The model under review builds one solid part; all positions refer to its coordinate system, in mm. Face numbers are marked on the shaded views. Coordinates: 2 decimals unless noted, no trailing zeros. Order: outer loops, then holes, each group sorted by start corner. A loop starts at its lowest first (then second) coordinate and runs counter-clockwise, first axis right, second up. Notation, with made-up numbers: M -20.5,0.25 L -1.5,0.25 A32 ccw -1.5,38.25 Z; hole C 22.25,27.5 d5. An arc over 180 degrees is marked long. Answer in a Markdown table with one row per item.
from build123d import *

# Parameters (mm, degrees)
SKETCH1_R           = 3
BOSS_EXTRUDE2_DEPTH = 5


with BuildPart() as part:
    # Sketch1 → Boss-Extrude2 (new body)
    with BuildSketch(Plane(origin=(0, 0, 0), x_dir=(1, 0, 0), z_dir=(0, 1, 0))):
        with BuildLine():
            Line((-107.345005718, 88.870972468), (-6.913400561, -7.225295335))
            ThreePointArc((-6.913400561, -7.225295335), (0.220534203, -9.997567938), (7.225283293, -6.913413146))
            Line((7.225283293, -6.913413146), (99.173678137, 89.182854657))
            ThreePointArc((99.173678137, 89.182854657), (98.86180799, 103.321551097), (84.72311155, 103.009680949))
            Line((84.72311155, 103.009680949), (-0.311882189, 14.138683855))
            Line((-0.311882189, 14.138683855), (-93.518204595, 103.321563138))
            ThreePointArc((-93.518204595, 103.321563138), (-107.656900491, 103.009668365), (-107.345005718, 88.870972468))
        make_face()
        with Locations((-100.431605156, 96.096267803)):
            Circle(SKETCH1_R, mode=Mode.SUBTRACT)
        with Locations((91.948394844, 96.096267803)):
            Circle(SKETCH1_R, mode=Mode.SUBTRACT)
        Circle(SKETCH1_R, mode=Mode.SUBTRACT)
    extrude(amount=BOSS_EXTRUDE2_DEPTH)


solid = part.part
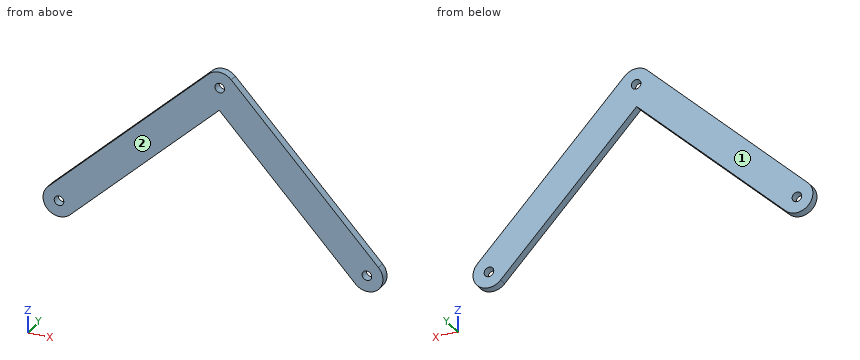
(1) The part is to be moulded in two halves that separate along Y. For the marked faces 1 and 2, say which applies: +Y half, -Y half, draft (parallel to the pull), parting line (faces both ways), or undercut.
Report:
| item | result |
|---|---|
| face 1 | +Y half |
| face 2 | -Y half |
(2) Take a section at C-C (z = -52.5). Write out the cut boundary in (x, y).
Report:
| item | result |
|---|---|
| outline | M -69.33,0 L -40.4,0 L -40.4,5 L -69.33,5 Z; M 36.39,0 L 64.07,0 L 64.07,5 L 36.39,5 Z |
(3) To check wall thickness, follow line 1 (X direction, y = 3.2, z = -98); line 2 (X direction, y = 3.25, z = -53); line 3 (X direction, y = 1.4, z = -59). State the ranges of each line that lie inside material, in increasing order. Write a range as [from, to].
Report:
| item | result |
|---|---|
| line 1 | [-110.25, -102.75], [-98.11, -87.96], [79.93, 89.63], [94.27, 101.77] |
| line 2 | [-69.86, -40.93], [36.87, 64.55] |
| line 3 | [-76.13, -47.2], [42.61, 70.29] |
(4) Take a section at D-D (x = -56.5). Write out the cut boundary in (y, z).
Report:
| item | result |
|---|---|
| outline | M 0,-67.9 L 5,-67.9 L 5,-40.22 L 0,-40.22 Z |
(5) Take a section at A-A (z = 0). Write out the cut boundary in (x, y).
Report:
| item | result |
|---|---|
| outline | M -14.46,0 L -3,0 L -3,5 L -14.46,5 Z; M 3,0 L 13.84,0 L 13.84,5 L 3,5 Z |
(6) Take a section at B-B (y = 2.3). Write out the cut boundary in (x, z) (3 decimals), then the cut area to 3 significant figures.
Report:
| item | result |
|---|---|
| outline | M -107.345,-88.871 A10 ccw -93.518,-103.322 L -0.312,-14.139 L 84.723,-103.01 A10 ccw 99.174,-89.183 L 7.225,6.913 A10 ccw -6.913,7.225 Z; hole C -100.432,-96.096 d6; hole C 0,0 d6; hole C 91.948,-96.096 d6 |
| area | 5,650 mm^2 |
(7) Insertion check: P1, Ø1.5, axis at x = 66, y = 1.5, coming from the +Z side; P2, Ø3.5, axis at x = 91.95, z = -96.1, coming from the -Y side. Each pin has a flat end and moves straight along its axis. Give the tip position at first contact, or say it passes through.
Report:
| item | result |
|---|---|
| P1 | z = -53.73 |
| P2 | through |
